Geometry: see drawing. Coordinates: mm, zero at the bounding-box minimum. A direction names the side the tool comes from. Give positions to 0.01 mm unless a question says otherwise; leave off trailing zeros. Loops run counter-clockwise (first coordinate to the right, second up) from the corner with the lowest first, then second, coordinate; pieces in that order, holes last. Notation, with made-up numbers: (53, 39.5) - (100, 39.5) arc R29 ccw to (100, 61.5) - close; hole circle Ø3 at (53.25, 71). An arc over 180 degrees is marked (long way). Use CSV: the item, a comma, the result in double quotes. Start each with the question number.
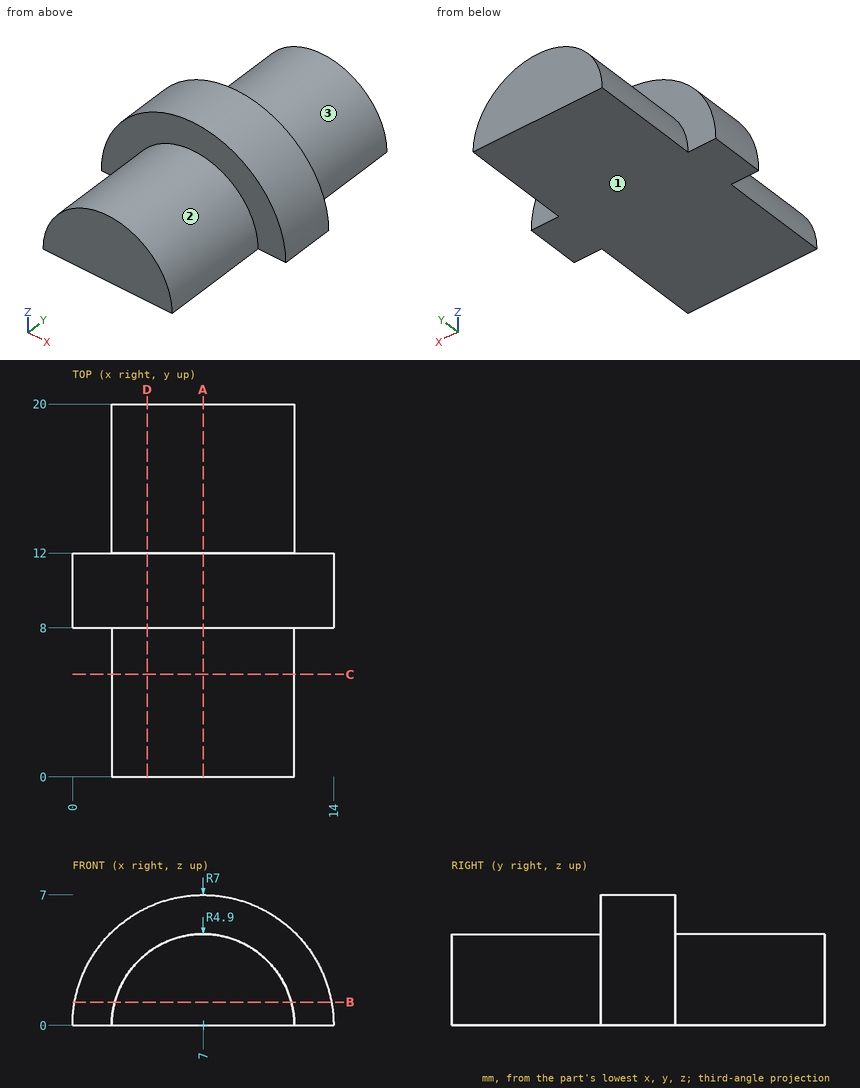
Item 1: Ray query, probe 1 along Y at (x, z) = (13.5, 0.75); probe 2 along Z at (x, y) = (8.25, 6.25); probe 3 along X at (y, z) = (8.25, 4). Return the intervals inside material, ascending.
Item 2: Reachability of the marked faces 1, 2 and 3 from +Z, -Z, +X, -X, +Y, -Y: full face, straight path, thin tool, end or side. Return the list, or none.
Item 3: Section A-A (x = 7). Output: boundary loops of the cut face in (y, z), plus the area to 3 significant figures.
Item 4: Section D-D (x = 4). Output: boundary loops of the cut face in (y, z).
Item 5: Section B-B (z = 1.25). Output: boundary loops of the cut face in (x, y), plus the area to 3 significant figures.
Item 6: Pin query (flat end, axial travel): pin 1 Ø4 at (x, z) = (10, 4) entering from +Y; pin 2 Ø2 at (y, z) = (10.5, 5) entering from -X. Return the tip coordinate at first contact, or that it passes through.
Item 7: Section C-C (y = 5.5). Output: boundary loops of the cut face in (x, z), plus the area to 3 significant figures.
Outcome:
1,probe 1,"y = 8 to 12"
1,probe 2,"z = 0 to 4.74"
1,probe 3,"x = 1.26 to 12.74"
2,face 1,"-Z, +X, -X, +Y, -Y"
2,face 2,"+Z, -Y"
2,face 3,"+Z, +Y"
3,outline,"(0, 0) - (20, 0) - (20, 4.9) - (12, 4.9) - (12, 7) - (8, 7) - (8, 4.9) - (0, 4.9) - close"
3,area,"106 mm2"
4,outline,"(0, 0) - (20, 0) - (20, 3.87) - (12, 3.87) - (12, 6.32) - (8, 6.32) - (8, 3.87) - (0, 3.87) - close"
5,outline,"(0.11, 8) - (2.26, 8) - (2.26, 0) - (11.74, 0) - (11.74, 8) - (13.89, 8) - (13.89, 12) - (11.74, 12) - (11.74, 20) - (2.26, 20) - (2.26, 12) - (0.11, 12) - close"
5,area,"207 mm2"
6,pin 1,"stops at y = 20"
6,pin 2,"stops at x = 1.26"
7,outline,"(2.1, 0) - (11.9, 0) arc R4.9 ccw to start"
7,area,"37.7 mm2"
